Check sheet for the drawn part. Datum: minimum x, y, z corner. Units: mm. A direction names the side the tool comes from. Coordinates: 2 decimals unless noted, no trailing zeros. Loops run counter-clockwise (first coordinate to the right, second up) from the corner with the lowest first, then second, coordinate; pieces in that order, holes last. Notation, with made-up numbers: (55.5, 86) - (108.5, 86) arc R22 cw to (108.5, 112) - close; hole circle Ø9 at (-10, 50.25). An arc over 180 degrees is marked (long way). Answer as CSV lines item,"result". Start each with the question number.
1. Cross-section at B-B (x = 18.5). Enter the section's corners in (y, z).
2. Release check for a two-part mould opening along X. For the marked faces 1, 2, 3 and 4 record: pulls with the +X half, pulls with the -X half, needs draft (parallel to the pull), parting line crosses it, or undercut.
3. Material ranges on line 1 (X direction, y = 4, z = 11.75); line 2 (Y direction, x = 7.25, z = 15.5); line 3 (X direction, y = 1.75, z = 6.75), recorded low to high. Write a range as [from, to].
4. Gauge pin test, flat ends, axial feed: P1, Ø4, axis at x = 18, z = 11, coming from the -Y side; P2, Ø0.5, axis at x = 4.5, z = 5.5, coming from the -Y side; P3, Ø2.5, axis at x = 18, z = 11, coming from the -Y side. Record the tip position at first contact, or that the pin passes through.
5. Cross-section at A-A (z = 4). Enter the section's corners in (x, y), plus the area to 3 significant figures.
6. Set-up check for the marked faces 5, 6, 7, 8 and 9: record each of +Z, -Z, +X, -X, +Y, -Y from which the full face is reachable in a straight line by a thin tool's end or side.
7. Cross-section at C-C (y = 7.25). Enter the section's corners in (x, z).
8. Cross-section at D-D (x = 9). Enter the section's corners in (y, z).
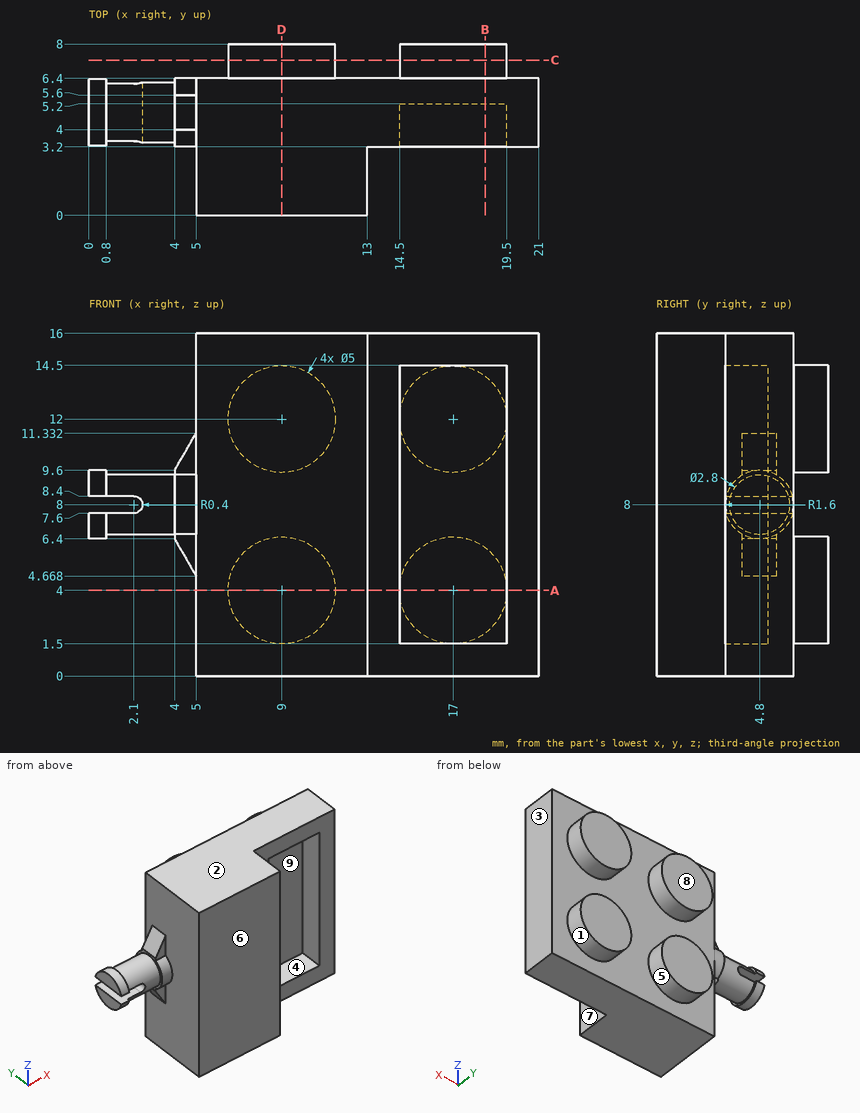
Values follow:
1,outline,"(3.2, 0) - (6.4, 0) - (6.4, 2) - (8, 2) - (8, 6) - (6.4, 6) - (6.4, 10) - (8, 10) - (8, 14) - (6.4, 14) - (6.4, 16) - (3.2, 16) - (3.2, 14.5) - (5.2, 14.5) - (5.2, 1.5) - (3.2, 1.5) - close"
2,face 1,"undercut"
2,face 2,"needs draft"
2,face 3,"pulls with the +X half"
2,face 4,"undercut"
3,line 1,"x = [5, 14.5], [19.5, 21]"
3,line 2,"y = [0, 6.4]"
3,line 3,"x = [5, 13]"
4,P1,"stops at y = 3.2"
4,P2,"stops at y = 4"
4,P3,"stops at y = 5.2"
5,outline,"(5, 0) - (13, 0) - (13, 3.2) - (14.5, 3.2) - (14.5, 5.2) - (19.5, 5.2) - (19.5, 3.2) - (21, 3.2) - (21, 6.4) - (19.5, 6.4) - (19.5, 8) - (14.5, 8) - (14.5, 6.4) - (11.5, 6.4) - (11.5, 8) - (6.5, 8) - (6.5, 6.4) - (5, 6.4) - close"
5,area,"82.8 mm²"
6,face 5,"+Y"
6,face 6,"+Z, -Z, +X, -X, -Y"
6,face 7,"+Z, -Z, +X, -Y"
6,face 8,"+Z, -Z, +X, -X, +Y"
6,face 9,"-Y"
7,outline,"circle Ø5 at (9, 4); circle Ø5 at (9, 12); circle Ø5 at (17, 4); circle Ø5 at (17, 12)"
8,outline,"(0, 0) - (6.4, 0) - (6.4, 1.5) - (8, 1.5) - (8, 6.5) - (6.4, 6.5) - (6.4, 9.5) - (8, 9.5) - (8, 14.5) - (6.4, 14.5) - (6.4, 16) - (0, 16) - close"
